Design review of the part built by this model. Coordinates are the model's own, in mm. A direction names the side the tool comes from. Round coordinates to 2 decimals unless told otherwise and drop trailing zeros. Loops run counter-clockwise (first coordinate to the right, second up) from the corner with the lowest first, then second, coordinate; pieces in that order, holes last. Notation, with made-up numbers: (81.25, 87.25) - (136.25, 87.25) arc R26 cw to (136.25, 107.25) - close; hole circle Ø1 at (-15.5, 74). An arc over 180 degrees is marked (long way). Answer as CSV lines item,"result". Start each with the question number.
(1) For faces 5 (the cylindrical face through (-0.766, 1.479, 36.347)), 6 (the flat face through (0, 3, -12)), list the 3-axis set-ups (+Z, -Z, +X, -X, +Y, -Y) from which the entire face can be reached by the end or side of a thin tool; tool diameter is ignored.
(2) Consider section D-D (z = -42.5). Give the boundary of the cut face in (x, y), and give its area (3 significant figures).
(3) Mouldability with a two-part tool opening along Y and no side actions: class faces 1 (the cylindrical face through (4, 1, -44)), 2 (the cylindrical face through (0, 41, 66)), 3 (the cylindrical face through (-14.1, 31.51, 66.02)), 4 (the flat face through (0, 0, -12)) as released by +Y, released by -Y, zero draft, split by the parting line, or undercut.
(4) Wall thickness on L1, parallel to X at y = 1.7, z = -59.5; L2, parallel to X at y = 30, z = 66; L3, parallel to Y at x = 2.5, z = 11.5: over which ranges is each line inside the solid? List them lowest first.
(5) Consider section A-A (z = -59.5). Give the boundary of the cut face in (x, y).
(6) For P1, Ø2.5, axis at x = -12.99, y = 30.5, coming from the +Z side; P2, Ø5, axis at x = -8, z = -67.5, coming from the +Y side; P3, Ø5, axis at x = 0, z = 34.5, coming from the -Y side; P4, Ø4, axis at x = -1.5, y = 35.5, coming from the -Z side, all flat-tipped, find the tip position at first contact; note any pin that passes through.
(7) Consider section C-C (y = 14). Give the boundary of the cut face in (x, z), and give its area (3 significant figures).
(8) Consider section B-B (x = 0). Count the separate pieces of the cut face and the enclosed holes in it, and give its area (3 significant figures).
from build123d import *

# Parameters (mm, degrees)
SKETCH_1_R          = 1.5
SKETCH_1_R_2        = 2.5
SKETCH_1_R_3        = 2
EXTRUDE_1_DEPTH     = 3
SKETCH_2_W          = 36
SKETCH_2_H          = 3
EXTRUDE_2_DEPTH     = 41
CUT_EXTRUDE_1_DEPTH = 4
SKETCH_5_R          = 1.5
SKETCH_5_R_2        = 12
CUT_EXTRUDE_2_DEPTH = 4
FILLET_1_R          = 3
FILLET_2_R          = 1


with BuildPart() as part:
    # 草图1 → 凸台-拉伸1 (new body)
    with BuildSketch(Plane(origin=(0, 0, 0), x_dir=(1, 0, 0), z_dir=(0, 1, 0))):
        with BuildLine():
            Line((18, -67.5), (-18, -67.5))
            Line((-18, -67.5), (-18, 67.5))
            ThreePointArc((-18, 67.5), (0, 85.5), (18, 67.5))
            Line((18, 67.5), (18, -67.5))
        make_face()
        with Locations(Location((0, 75.5, 0), (0, 0, 270))):
            Circle(SKETCH_1_R, mode=Mode.SUBTRACT)
        with Locations(Location((0, 59.5, 0), (0, 0, 270))):
            Circle(SKETCH_1_R, mode=Mode.SUBTRACT)
        with Locations(Location((-8, 67.5, 0), (0, 0, 270))):
            Circle(SKETCH_1_R, mode=Mode.SUBTRACT)
        with Locations(Location((8, 67.5, 0), (0, 0, 270))):
            Circle(SKETCH_1_R, mode=Mode.SUBTRACT)
        with Locations(Location((0, 67.5, 0), (0, 0, 270))):
            Circle(SKETCH_1_R_2, mode=Mode.SUBTRACT)
        with Locations(Location((-4, 42.5, 0), (0, 0, 270))):
            Circle(SKETCH_1_R, mode=Mode.SUBTRACT)
        with Locations(Location((4, 42.5, 0), (0, 0, 270))):
            Circle(SKETCH_1_R, mode=Mode.SUBTRACT)
        with Locations(Location((0, -34.5, 0), (0, 0, 270))):
            Circle(SKETCH_1_R_3, mode=Mode.SUBTRACT)
    extrude(amount=EXTRUDE_1_DEPTH)

    # 草图2 → 凸台-拉伸2 (add)
    with BuildSketch(Plane(origin=(0, 3, 0), x_dir=(1, 0, 0), z_dir=(0, 1, 0))):
        with Locations((0, -66)):
            Rectangle(SKETCH_2_W, SKETCH_2_H)
    extrude(amount=EXTRUDE_2_DEPTH)

    # 草图3 → 切除-拉伸1 (cut)
    with BuildSketch(Plane.XY.offset(67.5)):
        with BuildLine():
            Line((-18, 44), (-18, 23))
            ThreePointArc((-18, 23), (0, 41), (18, 23))
            Line((18, 23), (18, 44))
            Line((18, 44), (-18, 44))
        make_face()
    extrude(amount=-CUT_EXTRUDE_1_DEPTH, mode=Mode.SUBTRACT)

    # 草图5 → 切除-拉伸2 (cut)
    with BuildSketch(Plane.XY.offset(67.5)):
        with Locations((0, 8)):
            Circle(SKETCH_5_R)
        with Locations((-12.990381057, 30.5)):
            Circle(SKETCH_5_R)
        with Locations((12.990381057, 30.5)):
            Circle(SKETCH_5_R)
        with Locations((0, 23)):
            Circle(SKETCH_5_R_2)
    extrude(amount=-CUT_EXTRUDE_2_DEPTH, mode=Mode.SUBTRACT)

    # 圆角1
    fillet_1_edges = [part.edges().sort_by_distance(p)[0] for p in [
        (0, 0, 67.5),
    ]]
    fillet(fillet_1_edges, radius=FILLET_1_R)

    # 圆角2
    fillet_2_edges = [part.edges().sort_by_distance(p)[0] for p in [
        (0, 3, 64.5),
    ]]
    fillet(fillet_2_edges, radius=FILLET_2_R)


solid = part.part
Determined:
1,face 5,"+Y, -Y"
1,face 6,"-Z, +X, -X, +Y"
2,outline,"(-18, 0) - (-5.5, 0) - (-5.5, 3) - (-18, 3) - close; (-2.5, 0) - (2.5, 0) - (2.5, 3) - (-2.5, 3) - close; (5.5, 0) - (18, 0) - (18, 3) - (5.5, 3) - close"
2,area,"90.0 mm^2"
3,face 1,"zero draft"
3,face 2,"released by +Y"
3,face 3,"undercut"
3,face 4,"released by -Y"
4,L1,"x = -18 to -1.5, 1.5 to 18"
4,L2,"x = -16.58 to -14.4, -11.58 to -9.75, 9.75 to 11.58, 14.4 to 16.58"
4,L3,"y = 0 to 3"
5,outline,"(-18, 0) - (-1.5, 0) - (-1.5, 3) - (-18, 3) - close; (1.5, 0) - (18, 0) - (18, 3) - (1.5, 3) - close"
6,P1,"passes through"
6,P2,"stops at y = 3"
6,P3,"stops at y = 0"
6,P4,"stops at z = 64.5"
7,outline,"(-18, 64.5) - (-7.94, 64.5) - (-7.94, 67.5) - (-18, 67.5) - close; (7.94, 64.5) - (18, 64.5) - (18, 67.5) - (7.94, 67.5) - close"
7,area,"60.4 mm^2"
8,separate pieces,"7"
8,enclosed holes,"0"
8,area,"445 mm^2"
